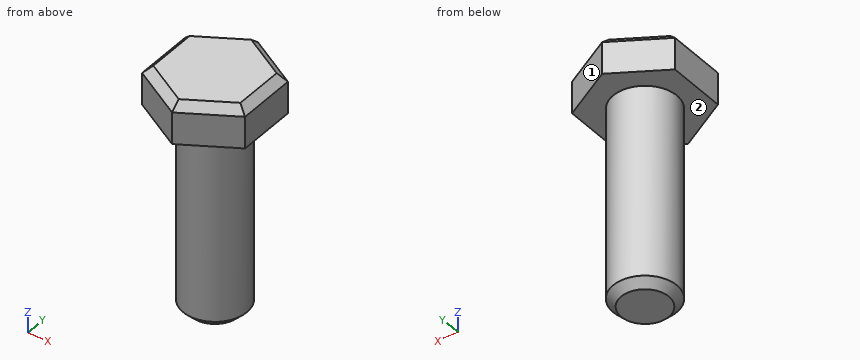
```python
from build123d import *

# Parameters (mm, degrees)
F1_DEPTH = 5
F2_R     = 4
F3_DEPTH = 25
F4_SIZE  = 1
F5_SIZE  = 1


with BuildPart() as f1:
    # F0 (on Top) → F1 (new body)
    with BuildSketch(Plane.XY):
        Polygon((-0.013194, -7.479013), (6.470418, -3.750933), (6.483613, 3.72808), (0.013194, 7.479013), (-6.470418, 3.750933), (-6.483613, -3.72808), align=None)
    extrude(amount=F1_DEPTH)

    # F2 (on Top) → F3 (join)
    with BuildSketch(Plane.XY):
        Circle(F2_R)
    extrude(amount=-F3_DEPTH)

    # F4
    f4_edges = [f1.edges().sort_by_distance(p)[0] for p in [
        (-4, 0, -25),
    ]]
    chamfer(f4_edges, length=F4_SIZE)

    # F5
    f5_edges = [f1.edges().sort_by_distance(p)[0] for p in [
        (6.477015, -0.011427, 5),
        (3.228612, -5.614973, 5),
        (3.248403, 5.603547, 5),
        (-6.477015, 0.011427, 5),
        (-3.248403, -5.603547, 5),
        (-3.228612, 5.614973, 5),
    ]]
    chamfer(f5_edges, length=F5_SIZE)


solid = f1.part
```
Here's how the part is built. I have some questions about the finished solid (model axes, mm). Face numbers are marked on the shaded views. A direction names the side the tool comes from. Coordinates: 2 decimals unless noted, no trailing zeros. Order: outer loops, then holes, each group sorted by start corner. A loop starts at its lowest first (then second) coordinate and runs counter-clockwise, first axis right, second up. Notation, with made-up numbers: (-23.75, 58) -> (25.25, 58) arc R37 ccw to (25.25, 94) -> close; hole circle Ø4 at (37.5, 52.5). An arc over 180 degrees is marked (long way). Return JSON: item names as keys, results as strings.
1) If I drill on probe 1 along Z at (x, y) = (1.5, -4); probe 2 along Z at (x, y) = (-4, 4.75); probe 3 along X at (y, z) = (0.25, -9), over which ranges is the centre line in solid material (lowest first)?
Conclusion:
{"probe 1": "z = 0 to 5", "probe 2": "z = 0 to 4.37", "probe 3": "x = -3.99 to 3.99"}
2) If we section it at B-B on y = 0: List the corners of the cut face in (x, z) for me.
Conclusion:
{"outline": "(-6.48, 0) -> (-4, 0) -> (-4, -24) -> (-3, -25) -> (3, -25) -> (4, -24) -> (4, 0) -> (6.48, 0) -> (6.48, 4) -> (5.48, 5) -> (-5.48, 5) -> (-6.48, 4) -> close"}
3) If we section it at A-A on z = 3.25: List the corners of the cut face in (x, y) for me, plus the area to 3 significant figures.
Conclusion:
{"outline": "(-6.48, -3.73) -> (-0.01, -7.48) -> (6.47, -3.75) -> (6.48, 3.73) -> (0.01, 7.48) -> (-6.47, 3.75) -> close", "area": "145 mm²"}
4) I'm going to push flat-ended pins straight in: P1, Ø1.5, axis at x = -0.5, z = -6, coming from the +Y side; P2, Ø5, axis at x = -1.5, z = -11, coming from the -Y side; P3, Ø5, axis at x = -3.5, z = -14.5, coming from the +Y side. Where does each tip first touch, or does it pass through?
Conclusion:
{"P1": "stops at y = 4", "P2": "stops at y = -4", "P3": "stops at y = 3.87"}
5) On a 3-axis mill with a long thin cutter (end or side, diameter ignored), from which of +Z, -Z, +X, -X, +Y, -Y can I reach the whole of each face in a straight line? I mean the marked faces 1 and 2. Say none if no direction works.
Conclusion:
{"face 1": "+Z, -Z, +X, +Y", "face 2": "-Z"}
6) If we section it at C-C on x = -4.5: List the corners of the cut face in (y, z) for me, plus the area to 3 significant figures.
Conclusion:
{"outline": "(-4.88, 0) -> (4.88, 0) -> (4.88, 4) -> (3.73, 5) -> (-3.72, 5) -> (-4.88, 4) -> close", "area": "47.7 mm²"}
7) If we section it at D-D on z = -10: List the corners of the cut face in (x, y) for me.
Conclusion:
{"outline": "circle Ø8 at (0, 0)"}
